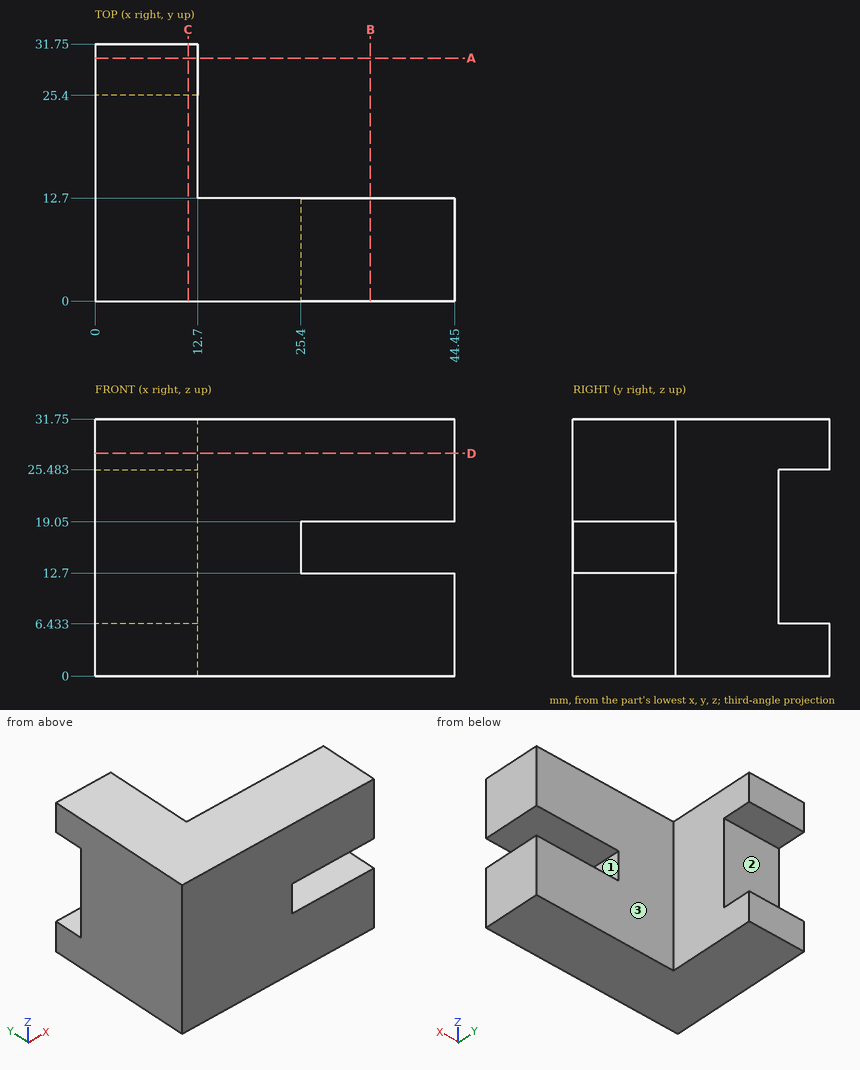
Print and shaded views of the part. All mm, measured from the part's lowest x, y and z. A direction names the side the tool comes from. Round coordinates to 2 decimals unless told otherwise and drop trailing zeros. Order: outer loops, then holes, each group sorted by start corner. A loop starts at its lowest first (then second) coordinate and runs counter-clockwise, first axis right, second up. Notation, with made-up numbers: (45, 13.5) - (104, 13.5) arc R13 cw to (104, 36.5) - close; hole circle Ø4 at (53.25, 78.25). An arc over 180 degrees is marked (long way). Use a Markdown table: item, result.
1) Saw through at C-C on x = 11.5. Write the cut outline in (y, z), and give its area (3 significant figures).
Recorded:
| item | result |
|---|---|
| outline | (0, 0) - (31.75, 0) - (31.75, 6.43) - (25.4, 6.43) - (25.4, 25.48) - (31.75, 25.48) - (31.75, 31.75) - (0, 31.75) - close |
| area | 887 mm² |
2) Flat gauge pins, fed straight in: pin 1 Ø3 at (x, z) = (31, 22.5) entering from +Y; pin 2 Ø9.5 at (y, z) = (21, 15.5) entering from +X; pin 3 Ø14 at (x, z) = (5, 16) entering from +Y. Where does each tip first touch, or does it go through?
Recorded:
| item | result |
|---|---|
| pin 1 | stops at y = 12.7 |
| pin 2 | stops at x = 12.7 |
| pin 3 | stops at y = 25.4 |
3) Wall check: L1, parallel to Z at x = 2, y = 30; L2, parallel to X at y = 22, z = 12.5. Give the ranges that are in metal, low to high.
Recorded:
| item | result |
|---|---|
| L1 | z = 0 to 6.43, 25.48 to 31.75 |
| L2 | x = 0 to 12.7 |
4) Saw through at D-D on z = 27.5. Write the cut outline in (x, y).
Recorded:
| item | result |
|---|---|
| outline | (0, 0) - (44.45, 0) - (44.45, 12.7) - (12.7, 12.7) - (12.7, 31.75) - (0, 31.75) - close |
5) Tool access for the marked faces 1, 2 and 3: list every direction of +Z, -Z, +X, -X, +Y, -Y with a clear straight run to the whole face (end or side of a thin tool).
Recorded:
| item | result |
|---|---|
| face 1 | +X, +Y, -Y |
| face 2 | +X, -X, +Y |
| face 3 | +Z, -Z, +X, +Y |
6) Saw through at A-A on y = 30. Write the cut outline in (x, z), and give its area (3 significant figures).
Recorded:
| item | result |
|---|---|
| outline | (0, 0) - (12.7, 0) - (12.7, 6.43) - (0, 6.43) - close; (0, 25.48) - (12.7, 25.48) - (12.7, 31.75) - (0, 31.75) - close |
| area | 161 mm² |
7) Saw through at B-B on x = 34. Write the cut outline in (y, z).
Recorded:
| item | result |
|---|---|
| outline | (0, 0) - (12.7, 0) - (12.7, 12.7) - (0, 12.7) - close; (0, 19.05) - (12.7, 19.05) - (12.7, 31.75) - (0, 31.75) - close |
